from build123d import *

# Parameters (mm, degrees)
F0_W     = 305
F0_H     = 440
F1_DEPTH = 305
F3_D     = 20.25
F4_W     = 50
F4_H     = 100
F5_DEPTH = 440
F6_DEPTH = 440


with BuildPart() as f1:
    # F0 (on Front) → F1 (new body)
    with BuildSketch(Plane.XZ):
        with Locations((152.5, 2.728686)):
            Rectangle(F0_W, F0_H)
    extrude(amount=F1_DEPTH)

    # F3 (through all)
    with Locations(Plane.XY.offset(222.728686)):
        with Locations((152.5, -24.5)):
            Hole(F3_D / 2)

    # F4 (on face) → F5 (join)
    with BuildSketch(Plane(origin=(0, 0, -217.271314), x_dir=(1, 0, 0), z_dir=(0, 0, -1))):
        with Locations((25, 255)):
            Rectangle(F4_W, F4_H)
    extrude(amount=F5_DEPTH)

    # F4 (on face) → F6 (join)
    with BuildSketch(Plane(origin=(0, 0, -217.271314), x_dir=(1, 0, 0), z_dir=(0, 0, -1))):
        with Locations((280, 255)):
            Rectangle(F4_W, F4_H)
        with Locations((280, 50)):
            Rectangle(F4_W, F4_H)
        with Locations((25, 50)):
            Rectangle(F4_W, F4_H)
    extrude(amount=F6_DEPTH)


solid = f1.part
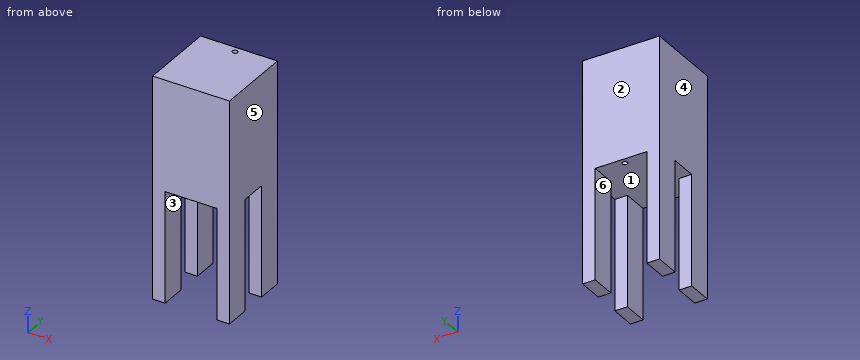
The listing builds one solid part. Answer for the finished solid, in the listing's coordinates (mm). Face numbers are marked on the shaded views. A direction names the side the tool comes from. Give positions to 0.01 mm unless a question says otherwise; leave off trailing zeros. Write each loop counter-clockwise with the first axis right and the second up, starting at its lowest first coordinate (ties: lowest second). Pieces come first, ordered by that corner, then holes. Notation, with made-up numbers: (40, -9.5) -> (83, -9.5) arc R5 cw to (83, -0.5) -> close; hole circle Ø3 at (16, 52.5). An arc over 180 degrees is marked (long way). One line per question, with ' | ' between items. Start each with the question number.
1. For the marked faces 5 and 6, determine the directions among +Z, -Z, +X, -X, +Y, -Y from which every point of the face is accessible in a straight line to the end or side of a thin tool.
2. Section B-B (y = -24.5) is taken. Determine the outline of the cut face in (x, z) (3 decimals).
3. Section A-A (x = 152.5) is taken. Determine the outline of the cut face in (y, z) (3 decimals).
4. Section D-D (y = -240) is taken. Determine the outline of the cut face in (x, z), plus the area to 3 significant figures.
5. Given pin 1 Ø8 at (x, y) = (90.5, -239.5) entering from -Z, flat-ended and moving along its own axis, determine where the tip first touches the part or whether it passes through.
6. Section C-C (z = -544) is taken. Determine the outline of the cut face in (x, y), plus the area to 3 significant figures.
7. For a pull along X with two mould halves and no side action, classify the marked faces 1, 2, 3 and 4 as pulls with the +X half, pulls with the -X half, needs draft (parallel to the pull), parting line crosses it, or undercut.
8. Find the intervals of material crossed by probe 1 along X at (y, z) = (-24, 101); probe 2 along Y at (x, z) = (152.5, 31.5) (3 decimals); probe 3 along X at (y, z) = (-99.5, -612), in increasing order.
Response values:
1) face 5: +Z, -Z, +X, +Y, -Y | face 6: -Z, +Y, -Y
2) outline: (0, -657.271) -> (50, -657.271) -> (50, -217.271) -> (142.375, -217.271) -> (142.375, 222.729) -> (0, 222.729) -> close; (162.625, -217.271) -> (255, -217.271) -> (255, -657.271) -> (305, -657.271) -> (305, 222.729) -> (162.625, 222.729) -> close
3) outline: (-305, -217.271) -> (-34.625, -217.271) -> (-34.625, 222.729) -> (-305, 222.729) -> close; (-14.375, -217.271) -> (0, -217.271) -> (0, 222.729) -> (-14.375, 222.729) -> close
4) outline: (0, -657.27) -> (50, -657.27) -> (50, -217.27) -> (255, -217.27) -> (255, -657.27) -> (305, -657.27) -> (305, 222.73) -> (0, 222.73) -> close | area: 178,000 mm2
5) pin 1: z = -217.27
6) outline: (0, -305) -> (50, -305) -> (50, -205) -> (0, -205) -> close; (0, -100) -> (50, -100) -> (50, 0) -> (0, 0) -> close; (255, -305) -> (305, -305) -> (305, -205) -> (255, -205) -> close; (255, -100) -> (305, -100) -> (305, 0) -> (255, 0) -> close | area: 20,000 mm2
7) face 1: undercut | face 2: needs draft | face 3: undercut | face 4: pulls with the -X half
8) probe 1: 0 to 142.39, 162.61 to 305 | probe 2: -305 to -34.625, -14.375 to 0 | probe 3: 0 to 50, 255 to 305
